Work out the finished part from the listing and answer in its coordinate system (mm). Face numbers are marked on the shaded views. A direction names the side the tool comes from. Coordinates: 2 decimals unless noted, no trailing zeros. Loops run counter-clockwise (first coordinate to the right, second up) from the corner with the lowest first, then second, coordinate; pieces in that order, holes last. Notation, with made-up numbers: (-39, -13) - (-31, -13) arc R16 cw to (-31, 12) - close; hole circle Ø1 at (88.25, -23). An arc over 180 degrees is marked (long way). Write each question's results on one line, items separated by ' | '. Start each with the question number.
1. A cutting plane is placed at B-B on y = -8. Determine the outline of the cut face in (x, z), then the cut area to 4 significant figures.
2. Find the intervals of material crossed by line 1 along Z through (x, y) = (4, -8); line 2 along Z through (x, y) = (-10.5, -14); line 3 along Y through (x, z) = (12, 65.5), in increasing order. Write a range as [from, to].
3. A cutting plane is placed at C-C on z = 56.5. Determine the outline of the cut face in (x, y), then the cut area to 3 significant figures.
4. Determine the mould class of the marked faces 1, 2 and 3 for opening direction Y: released by +Y, released by -Y, zero draft, split by the parting line, or undercut.
5. A cutting plane is placed at D-D on y = 27.5. Determine the outline of the cut face in (x, z).
6. A cutting plane is placed at A-A on z = 81. Determine the outline of the cut face in (x, y).
7. Which of the six approach directions +Z, -Z, +X, -X, +Y, -Y give full straight-line access (tool end or side, diameter ignored) to the marked faces 4, 5, 6, 7 and 8?
8. Each of these flat-tipped pins is pushed along its axis until it touches: P1, Ø6, axis at x = 19, z = 53, coming from the -Y side; P2, Ø5, axis at x = 23, z = 31.5, coming from the +Y side; P3, Ø1.5, axis at x = -18, z = 84, coming from the +Y side. Where does it stop, or does it pass through?
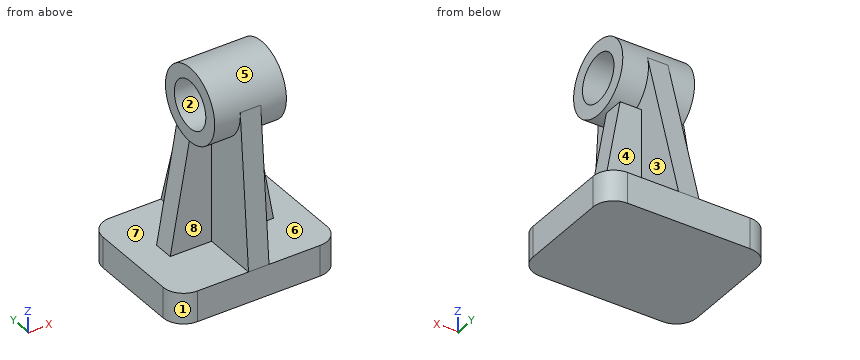
from build123d import *

# Parameters (mm, degrees)
SKETCH1_W           = 64
SKETCH1_H           = 80
BOSS_EXTRUDE1_DEPTH = 15
FILLET2_R           = 10
SKETCH2_R           = 18
SKETCH2_R_2         = 11.5
EXTRUDE_THIN1_DEPTH = 17.5
BOSS_EXTRUDE2_DEPTH = 5
BOSS_EXTRUDE3_DEPTH = 5


with BuildPart() as part:
    # Sketch1 → Boss-Extrude1 (new body)
    with BuildSketch(Plane(origin=(0, 0, 0), x_dir=(0, 1, 0), z_dir=(0, 0, 1))):
        Rectangle(SKETCH1_W, SKETCH1_H)
    extrude(amount=BOSS_EXTRUDE1_DEPTH)

    # Fillet2
    fillet2_edges = [part.edges().sort_by_distance(p)[0] for p in [
        (40, 32, 7.5),
        (40, -32, 7.5),
        (-40, -32, 7.5),
        (-40, 32, 7.5),
    ]]
    fillet(fillet2_edges, radius=FILLET2_R)



with BuildPart() as body_2:
    # Sketch2 → Extrude-Thin1 (new, symmetric)
    with BuildSketch(Plane.YZ):
        with Locations((-8, 88)):
            Circle(SKETCH2_R)
        with Locations((-8, 88)):
            Circle(SKETCH2_R_2, mode=Mode.SUBTRACT)
    extrude(amount=EXTRUDE_THIN1_DEPTH, both=True)


with BuildPart() as part_1:
    add(part.part)

    add(body_2.part)  # Boss-Extrude2 merges body 2
    # Sketch3 → Boss-Extrude2 (add, symmetric)
    with BuildSketch(Plane.YZ):
        with BuildLine():
            Line((-25.940694884, 89.459954482), (-32, 15))
            Line((-32, 15), (32, 15))
            Line((32, 15), (9.282478357, 93.03149499))
            ThreePointArc((9.282478357, 93.03149499), (9.819716755, 90.541199478), (10, 88))
            ThreePointArc((10, 88), (-8.730579254, 70.01483239), (-25.940694884, 89.459954482))
        make_face()
    extrude(amount=BOSS_EXTRUDE2_DEPTH, both=True)

    # Sketch4 → Boss-Extrude3 (add, symmetric)
    with BuildSketch(Plane(origin=(0, 0, 0), x_dir=(-1, 0, 0), z_dir=(0, 1, 0))):
        Polygon((-15.5, 70), (-25.197983939, 15), (25.197983939, 15), (15.5, 70), align=None)
    extrude(amount=BOSS_EXTRUDE3_DEPTH, both=True)


solid = part_1.part
Values:
1) outline: (-40, 0) - (40, 0) - (40, 15) - (5, 15) - (5, 70) - (17.5, 70) - (17.5, 76.5) - (-17.5, 76.5) - (-17.5, 70) - (-5, 70) - (-5, 15) - (-40, 15) - close; (-17.5, 99.5) - (17.5, 99.5) - (17.5, 106) - (-17.5, 106) - close | area: 2,205 mm^2
2) line 1: [0, 76.5], [99.5, 106] | line 2: [0, 15], [71.03, 78.19], [97.81, 104.97] | line 3: [-5, 5]
3) outline: (-17.88, -5) - (-5, -5) - (-5, -28.62) - (5, -28.62) - (5, -5) - (17.88, -5) - (17.88, 5) - (5, 5) - (5, 19.92) - (-5, 19.92) - (-5, 5) - (-17.88, 5) - close | area: 743 mm^2
4) face 1: released by -Y | face 2: undercut | face 3: zero draft
5) outline: (-38.35, 0) - (38.35, 0) - (38.35, 15) - (5, 15) - (5, 30.46) - (-5, 30.46) - (-5, 15) - (-38.35, 15) - close
6) outline: (-17.5, -24.58) - (-5, -24.58) - (-5, -26.63) - (5, -26.63) - (5, -24.58) - (17.5, -24.58) - (17.5, -17.12) - (-17.5, -17.12) - close; (-17.5, 1.12) - (17.5, 1.12) - (17.5, 8.58) - (5, 8.58) - (5, 12.79) - (-5, 12.79) - (-5, 8.58) - (-17.5, 8.58) - close
7) face 4: +X, +Y | face 5: none | face 6: +X | face 7: -X | face 8: -X, -Y
8) P1: y = -5 | P2: y = 5 | P3: y = 9.67
